The listing builds one solid part. Answer for the finished solid, in the listing's coordinates (mm). Face numbers are marked on the shaded views. A direction names the side the tool comes from. Give positions to 0.01 mm unless a question says otherwise; leave off trailing zeros. Order: outer loops, then holes, each group sorted by start corner. A loop starts at its lowest first (then second) coordinate and runs counter-clockwise, first axis right, second up. Notation, with made-up numbers: (-23.75, -33.75) - (2.25, -33.75) arc R14 cw to (2.25, -6.75) - close; hole circle Ø8 at (-30.5, 34.25). An arc over 180 degrees is marked (long way). Answer in a Markdown table with one row per item.
from build123d import *

# Parameters (mm, degrees)
F0_W     = 450
F0_H     = 420
F1_DEPTH = 800
F2_W     = 420
F2_H     = 630
F3_DEPTH = 385
F4_W     = 420
F4_H     = 5
F5_DEPTH = 344
F6_R     = 11.754652
F6_R_2   = 12.655136
F7_DEPTH = 10


with BuildPart() as f1:
    # F0 (on Top) → F1 (new body)
    with BuildSketch(Plane.XY):
        Rectangle(F0_W, F0_H)
    extrude(amount=F1_DEPTH)

    # F2 (on face) → F3 (cut)
    with BuildSketch(Plane.XZ.offset(210)):
        with Locations((0, 421.241939)):
            Rectangle(F2_W, F2_H)
    extrude(amount=-F3_DEPTH, mode=Mode.SUBTRACT)

    # F4 (on face) → F5 (join)
    with BuildSketch(Plane.XZ.offset(-175)):
        with Locations((0, 283.817353)):
            Rectangle(F4_W, F4_H)
    extrude(amount=F5_DEPTH)

    # F6 (on face) → F7 (join)
    with BuildSketch(Plane.XZ.offset(210)):
        with Locations((68.192616, 774.359405)):
            Circle(F6_R)
        with Locations((115.024745, 773.97877)):
            Circle(F6_R_2)
    extrude(amount=F7_DEPTH)


solid = f1.part
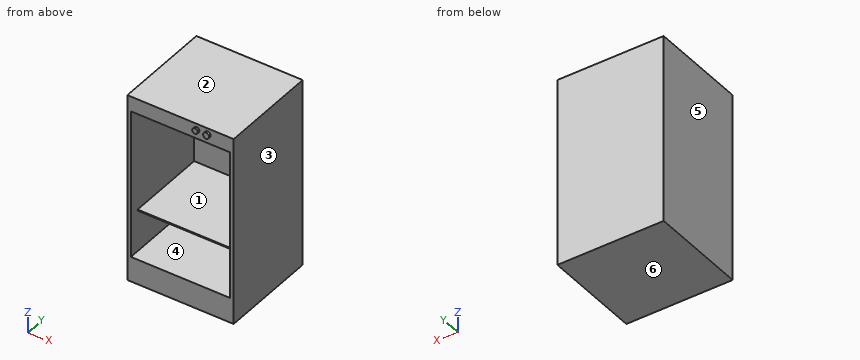
Item 1: Which of the six approach directions +Z, -Z, +X, -X, +Y, -Y give full straight-line access (tool end or side, diameter ignored) to the marked faces 1 and 2?
Answer block:
| item | result |
|---|---|
| face 1 | -Y |
| face 2 | +Z, +X, -X, +Y, -Y |
Item 2: Find section C-C on z = 415. Write down the section's boundary in (x, y), then the cut area to 3 significant figures.
Answer block:
| item | result |
|---|---|
| outline | (-225, -210) - (-210, -210) - (-210, 175) - (210, 175) - (210, -210) - (225, -210) - (225, 210) - (-225, 210) - close |
| area | 27,300 mm² |
Item 3: Consider line 1 (Z direction, x = 26.5, y = 153.5); line 2 (X direction, y = -29, z = 726.5); line 3 (Y direction, x = 53.5, z = 142). Determine where each line is inside the solid, lowest interval first.
Answer block:
| item | result |
|---|---|
| line 1 | 0 to 106.24, 281.32 to 286.32, 736.24 to 800 |
| line 2 | -225 to -210, 210 to 225 |
| line 3 | 175 to 210 |
Item 4: Each of these flat-tipped pins is pushed along its axis until it touches: P1, Ø12, axis at x = 99.5, z = 624, coming from the -Y side; P2, Ø4, axis at x = 56, z = 283, coming from the -Y side. Where does it stop, or does it pass through?
Answer block:
| item | result |
|---|---|
| P1 | y = 175 |
| P2 | y = -169 |
Item 5: Find section B-B on x = 165. Write down the section's boundary in (y, z), then the cut area to 3 significant figures.
Answer block:
| item | result |
|---|---|
| outline | (-210, 0) - (210, 0) - (210, 800) - (-210, 800) - (-210, 736.24) - (175, 736.24) - (175, 286.32) - (-169, 286.32) - (-169, 281.32) - (175, 281.32) - (175, 106.24) - (-210, 106.24) - close |
| area | 95,200 mm² |
Item 6: Find section A-A on y = -141.5. Write down the section's boundary in (x, z), then the cut area to 3 significant figures.
Answer block:
| item | result |
|---|---|
| outline | (-225, 0) - (225, 0) - (225, 800) - (-225, 800) - close; hole (-210, 106.24) - (210, 106.24) - (210, 281.32) - (-210, 281.32) - close; hole (-210, 286.32) - (210, 286.32) - (210, 736.24) - (-210, 736.24) - close |
| area | 97,500 mm² |
Item 7: Determine the mould class of the marked faces 3, 4, 5 and 6 for opening direction X: pulls with the +X half, pulls with the -X half, needs draft (parallel to the pull), parting line crosses it, or undercut.
Answer block:
| item | result |
|---|---|
| face 3 | pulls with the +X half |
| face 4 | undercut |
| face 5 | pulls with the -X half |
| face 6 | needs draft |
